from build123d import *

# Parameters (mm, degrees)
EXTRUDE_1_DEPTH          = 6.5
CUT_EXTRUDE_1_DEPTH      = 13.71573828
CUT_EXTRUDE_1_DEPTH_BACK = 13.71573828
SKETCH_2_W               = 3.7
SKETCH_2_H               = 1.2


with BuildPart() as part:
    # Эскиз1 → Бобышка-Вытянуть1 (new, symmetric)
    with BuildSketch(Plane(origin=(0, 0, 0), x_dir=(1, 0, 0), z_dir=(0, 1, 0))):
        with BuildLine():
            Line((-6.658312395, 0), (6.658312395, 0))
            ThreePointArc((6.658312395, 0), (6.996852653, -0.295417601), (6.75, -0.670843802))
            ThreePointArc((6.75, -0.670843802), (6.5, -1), (6.75, -1.329156198))
            ThreePointArc((6.75, -1.329156198), (6.996852653, -1.704582399), (6.658312395, -2))
            Line((6.658312395, -2), (8.955547022, -5.741842995))
            ThreePointArc((8.955547022, -5.741842995), (8.874693562, -6.143507105), (8.468237531, -6.091885079))
            Line((8.468237531, -6.091885079), (5.500699092, -2.534366135))
            ThreePointArc((5.500699092, -2.534366135), (4.718050783, -2.364111944), (4.360854377, -3.081004957))
            Line((4.360854377, -3.081004957), (4.893274759, -5.719437316))
            ThreePointArc((4.893274759, -5.719437316), (4.605767966, -6.185807283), (4.121027011, -5.930489228))
            Line((4.121027011, -5.930489228), (3.115902551, -3.038005813))
            ThreePointArc((3.115902551, -3.038005813), (2.415953046, -2.605439542), (1.849849185, -3.202573787))
            Line((1.849849185, -3.202573787), (1.650046399, -5.829228376))
            ThreePointArc((1.650046399, -5.829228376), (1.250599943, -6.199999551), (0.850046399, -5.830424668))
            Line((0.850046399, -5.830424668), (0.65, -3.300629586))
            ThreePointArc((0.65, -3.300629586), (0, -2.7), (-0.65, -3.300629586))
            Line((-0.65, -3.300629586), (-0.850046399, -5.830424668))
            ThreePointArc((-0.850046399, -5.830424668), (-1.250599943, -6.199999551), (-1.650046399, -5.829228376))
            Line((-1.650046399, -5.829228376), (-1.849849185, -3.202573787))
            ThreePointArc((-1.849849185, -3.202573787), (-2.415953046, -2.605439542), (-3.115902551, -3.038005813))
            Line((-3.115902551, -3.038005813), (-4.121027011, -5.930489228))
            ThreePointArc((-4.121027011, -5.930489228), (-4.605767966, -6.185807283), (-4.893274759, -5.719437316))
            Line((-4.893274759, -5.719437316), (-4.360854377, -3.081004957))
            ThreePointArc((-4.360854377, -3.081004957), (-4.718050783, -2.364111944), (-5.500699092, -2.534366135))
            Line((-5.500699092, -2.534366135), (-8.468237531, -6.091885079))
            ThreePointArc((-8.468237531, -6.091885079), (-8.874693562, -6.143507105), (-8.955547022, -5.741842995))
            Line((-8.955547022, -5.741842995), (-6.658312395, -2))
            ThreePointArc((-6.658312395, -2), (-6.996852653, -1.704582399), (-6.75, -1.329156198))
            ThreePointArc((-6.75, -1.329156198), (-6.5, -1), (-6.75, -0.670843802))
            ThreePointArc((-6.75, -0.670843802), (-6.996852653, -0.295417601), (-6.658312395, 0))
        make_face()
    extrude(amount=EXTRUDE_1_DEPTH, both=True)

    # Эскиз2 → Вырез-Вытянуть1 (cut, two sides: drawn at the far end of the back side and taken through both)
    with BuildSketch(Plane(origin=(0, 0, 0), x_dir=(0, 0, -1), z_dir=(1, 0, 0)).offset(-CUT_EXTRUDE_1_DEPTH_BACK)):
        with Locations((-4.35, -3.6)):
            Rectangle(SKETCH_2_W, SKETCH_2_H)
        with Locations((-4.35, 0)):
            Rectangle(SKETCH_2_W, SKETCH_2_H)
        with Locations((-4.35, 3.6)):
            Rectangle(SKETCH_2_W, SKETCH_2_H)
    extrude(amount=CUT_EXTRUDE_1_DEPTH + CUT_EXTRUDE_1_DEPTH_BACK, mode=Mode.SUBTRACT)


solid = part.part
Geometry: final body of the model. Coordinates: model frame, mm. A direction names the side the tool comes from. Round coordinates to 2 decimals unless told otherwise and drop trailing zeros. Order: outer loops, then holes, each group sorted by start corner. A loop starts at its lowest first (then second) coordinate and runs counter-clockwise, first axis right, second up.
Q1. Section D-D, the plane z = 1.75. Output: boundary loops of the cut face in (x, y), and give its area (3 significant figures).
Result sheet:
outline: (-6.99, -6.5) - (6.99, -6.5) - (6.99, 6.5) - (-6.99, 6.5) - close
area: 182 mm2
Q2. Pin query (flat end, axial travel): pin 1 (3 mm diameter, centred on y = 1.5, z = 2, fed in from +X); pin 2 (1.8 mm diameter, centred on x = 2, z = 4, fed in from -Y); pin 3 (0.6 mm diameter, centred on x = 6.5, y = 0, fed in from +Z); pin 4 (2 mm diameter, centred on y = -2.5, z = 4.5, fed in from -X). Return the tip coordinate at first contact, or that it passes through.
Result sheet:
pin 1: stops at x = 7.58
pin 2: stops at y = -6.5
pin 3: stops at z = 2.5
pin 4: stops at x = -8.81
Q3. Access query for faces 1 (the face through (6, -4, 2.5)), 2 (the face through (-1.75, -1.78, 4.53)). Directions: +Z, -Z, +X, -X, +Y, -Y. A direction counts if a zero-diameter tool reaches every point of the face in a straight line with its end or side. Return the directions, or none.
Result sheet:
face 1: +Z, +X, -X
face 2: +Z, +Y, -Y
Q4. Mould query, pull axis Z, two halves, no side actions, for faces 3 (the face through (4.623, 1.817, 4.382)), 4 (the face through (-6, -4, 2.5)), 5 (the face through (0, 0, 0)), 6 (the face through (1, -0.6, 4)). Classes: released by +Z, released by -Z, zero draft, split by the parting line, or undercut.
Result sheet:
face 3: undercut
face 4: released by +Z
face 5: released by -Z
face 6: zero draft
Q5. Section C-C, the plane z = 4. Give the number of separate pieces and of enclosed holes in the cut face, and give its area (3 significant figures).
Result sheet:
separate pieces: 24
enclosed holes: 0
area: 62.8 mm2
Q6. Material intervals for probe 1 along Y at (x, z) = (6.75, 3.75); probe 2 along X at (y, z) = (-5, 4); probe 3 along Z at (x, y) = (-1.25, 3.5), sorted ascending.
Result sheet:
probe 1: y = -6.5 to -4.2, -3 to -0.6, 0.6 to 3, 4.2 to 6.5
probe 2: x = -7.89 to -6.72, -4.55 to -3.45, -1.79 to -0.71, 0.71 to 1.79, 3.45 to 4.55, 6.72 to 7.89
probe 3: z = 0 to 2.5
Q7. Section B-B, the plane x = -6. Output: boundary loops of the cut face in (y, z).
Result sheet:
outline: (-6.5, 0) - (6.5, 0) - (6.5, 3.13) - (4.2, 3.13) - (4.2, 2.5) - (3, 2.5) - (3, 3.13) - (0.6, 3.13) - (0.6, 2.5) - (-0.6, 2.5) - (-0.6, 3.13) - (-3, 3.13) - (-3, 2.5) - (-4.2, 2.5) - (-4.2, 3.13) - (-6.5, 3.13) - close
